from build123d import *

# Parameters (mm, degrees)
SKETCH_W             = 62
SKETCH_H             = 28
SKETCH_W_2           = 58
SKETCH_H_2           = 24
PAD_DEPTH            = 10
SKETCH001_W          = 72
SKETCH001_H          = 38
SKETCH001_W_2        = 62
SKETCH001_H_2        = 28
PAD001_DEPTH         = 2
SKETCH002_R          = 1.15
POCKET_DEPTH         = 0.001
POCKET_DEPTH_BACK    = -10.001
SKETCH003_R          = 1.15
POCKET001_DEPTH      = 36.001
POCKET001_DEPTH_BACK = -36.001
FILLET_R             = 2


with BuildPart() as part:
    # Sketch → Pad (new body)
    with BuildSketch(Plane.XY):
        Rectangle(SKETCH_W, SKETCH_H)
        Rectangle(SKETCH_W_2, SKETCH_H_2, mode=Mode.SUBTRACT)
    extrude(amount=PAD_DEPTH)

    # Sketch001 → Pad001 (join)
    with BuildSketch(Plane.XY):
        Rectangle(SKETCH001_W, SKETCH001_H)
        Rectangle(SKETCH001_W_2, SKETCH001_H_2, mode=Mode.SUBTRACT)
    extrude(amount=PAD001_DEPTH)

    # Sketch002 → Pocket (cut, two sides)
    with BuildSketch(Plane.XY) as pocket_sk:
        with Locations((-33.5, 16.5)):
            Circle(SKETCH002_R)
        with Locations((33.5, 16.5)):
            Circle(SKETCH002_R)
        with Locations((33.5, -16.5)):
            Circle(SKETCH002_R)
        with Locations((-33.5, -16.5)):
            Circle(SKETCH002_R)
    extrude(amount=-POCKET_DEPTH, mode=Mode.SUBTRACT)
    extrude(pocket_sk.sketch, amount=-POCKET_DEPTH_BACK, mode=Mode.SUBTRACT)

    # Sketch003 → Pocket001 (cut, two sides)
    with BuildSketch(Plane.YZ) as pocket001_sk:
        with Locations((0, 6)):
            Circle(SKETCH003_R)
    extrude(amount=-POCKET001_DEPTH, mode=Mode.SUBTRACT)
    extrude(pocket001_sk.sketch, amount=-POCKET001_DEPTH_BACK, mode=Mode.SUBTRACT)

    # Fillet
    fillet_edges = [part.edges().sort_by_distance(p)[0] for p in [
        (-36, 19, 1),
        (-36, -19, 1),
        (36, -19, 1),
        (36, 19, 1),
        (31, 14, 6),
        (31, -14, 6),
        (-31, 14, 6),
        (-31, -14, 6),
    ]]
    fillet(fillet_edges, radius=FILLET_R)


solid = part.part
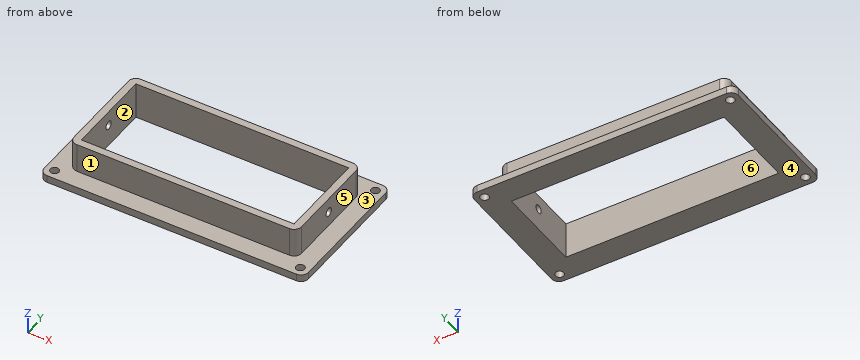
Can you work these out from the model? Positions are in its coordinate system, mm. Face numbers are marked on the shaded views. A direction names the side the tool comes from. Give positions to 0.01 mm unless a question says otherwise; leave off trailing zeros. Loops run counter-clockwise (first coordinate to the right, second up) from the corner with the lowest first, then second, coordinate; pieces in that order, holes last. Notation, with made-up numbers: (-27, -38.5) - (17, -38.5) arc R22 ccw to (17, -12.5) - close; hole circle Ø8 at (-29, -24.75). An arc over 180 degrees is marked (long way). Answer as a JSON object with one key per item and string values.
Q1. Which directions (+Z, -Z, +X, -X, +Y, -Y) give clear straight access to the entire face, cutting with the end or side of a thin tool? Please do the marked faces 4, 5 and 6.
Geometry says:
{"face 4": "-Z, +X, -X, +Y, -Y", "face 5": "+Z, +X, +Y, -Y", "face 6": "+Z, -Z"}
Q2. Imagine slicing it at C-C on x = -20. Write out the boundary of the cut face in (y, z).
Geometry says:
{"outline": "(-19, 0) - (-12, 0) - (-12, 10) - (-14, 10) - (-14, 2) - (-19, 2) - close; (12, 0) - (19, 0) - (19, 2) - (14, 2) - (14, 10) - (12, 10) - close"}
Q3. If I drill on L1, parallel to Y at x = -33.5, z = 0.8; L2, parallel to X at y = -16.5, z = 0.75; L3, parallel to Y at x = -16, z = 9, over which ranges is the centre line in solid material (lowest first)?
Geometry says:
{"L1": "-19 to -17.65, -15.35 to 15.35, 17.65 to 19", "L2": "-36 to -34.65, -32.35 to 32.35, 34.65 to 36", "L3": "-14 to -12, 12 to 14"}
Q4. Imagine slicing it at B-B on y = 0. Write out the boundary of the cut face in (x, z).
Geometry says:
{"outline": "(-36, 0) - (-29, 0) - (-29, 4.85) - (-31, 4.85) - (-31, 2) - (-36, 2) - close; (-31, 7.15) - (-29, 7.15) - (-29, 10) - (-31, 10) - close; (29, 0) - (36, 0) - (36, 2) - (31, 2) - (31, 4.85) - (29, 4.85) - close; (29, 7.15) - (31, 7.15) - (31, 10) - (29, 10) - close"}
Q5. If we mould it in two halves opening along Y, with no side actions, what happens to the marked faces 1, 2 and 3? For each: pulls with the +Y half, pulls with the -Y half, needs draft (parallel to the pull), parting line crosses it, or undercut.
Geometry says:
{"face 1": "pulls with the -Y half", "face 2": "undercut", "face 3": "needs draft"}
Q6. Will these pins go through, and if not, where does the flat tip stop? P1, Ø4, axis at y = 0.5, z = 5.5, coming from the +X side; P2, Ø3, axis at x = 33.5, y = 16.5, coming from the +Z side; P3, Ø2.5, axis at x = -12.5, z = 6, coming from the +Y side.
Geometry says:
{"P1": "x = 31", "P2": "z = 2", "P3": "y = 14"}
Q7. Imagine slicing it at A-A on y = 9.5. Write out the boundary of the cut face in (x, z), plus the area to 3 significant figures.
Geometry says:
{"outline": "(-36, 0) - (-29, 0) - (-29, 10) - (-31, 10) - (-31, 2) - (-36, 2) - close; (29, 0) - (36, 0) - (36, 2) - (31, 2) - (31, 10) - (29, 10) - close", "area": "60.0 mm²"}
Q8. Imagine slicing it at D-D on z = 3. Write out the boundary of the cut face in (x, y).
Geometry says:
{"outline": "(-31, -12) arc R2 ccw to (-29, -14) - (29, -14) arc R2 ccw to (31, -12) - (31, 12) arc R2 ccw to (29, 14) - (-29, 14) arc R2 ccw to (-31, 12) - close; hole (-29, -12) - (29, -12) - (29, 12) - (-29, 12) - close"}
